```python
from build123d import *

# Parameters (mm, degrees)
SKETCH1_R           = 32.5
BOSS_EXTRUDE1_DEPTH = 6
SKETCH16_R          = 1
CUT_EXTRUDE8_DEPTH  = 7
SKETCH17_R          = 2
CUT_EXTRUDE9_DEPTH  = 2.4
SKETCH18_R          = 4.5
CUT_EXTRUDE10_DEPTH = 7
SKETCH19_R          = 1.65
CUT_EXTRUDE11_DEPTH = 10
CUT_EXTRUDE12_DEPTH = 3
CUT_EXTRUDE13_DEPTH = 7


with BuildPart() as part:
    # Sketch1 → Boss-Extrude1 (new body)
    with BuildSketch(Plane.XY):
        Circle(SKETCH1_R)
    extrude(amount=BOSS_EXTRUDE1_DEPTH)

    # Sketch16 → Cut-Extrude8 (cut, through all)
    with BuildSketch(Plane.XY.offset(6)):
        with Locations((-8, 0)):
            Circle(SKETCH16_R)
        with Locations((-5.656854249, 5.656854249)):
            Circle(SKETCH16_R)
        with Locations((0, 8)):
            Circle(SKETCH16_R)
        with Locations((5.656854249, 5.656854249)):
            Circle(SKETCH16_R)
        with Locations((8, 0)):
            Circle(SKETCH16_R)
        with Locations((5.656854249, -5.656854249)):
            Circle(SKETCH16_R)
        with Locations((0, -8)):
            Circle(SKETCH16_R)
        with Locations((-5.656854249, -5.656854249)):
            Circle(SKETCH16_R)
    extrude(amount=-CUT_EXTRUDE8_DEPTH, mode=Mode.SUBTRACT)

    # Sketch17 → Cut-Extrude9 (cut)
    with BuildSketch(Plane.XY.offset(6)):
        with Locations((7.5, 0)):
            Circle(SKETCH17_R)
        with Locations((-8, 0)):
            Circle(SKETCH17_R)
        with Locations((0, -7.5)):
            Circle(SKETCH17_R)
        with Locations((0, 7.5)):
            Circle(SKETCH17_R)
        with Locations((-5.656854249, 5.656854249)):
            Circle(SKETCH17_R)
        with Locations((5.656854249, 5.656854249)):
            Circle(SKETCH17_R)
        with Locations((5.656854249, -5.656854249)):
            Circle(SKETCH17_R)
        with Locations((-5.656854249, -5.656854249)):
            Circle(SKETCH17_R)
    extrude(amount=-CUT_EXTRUDE9_DEPTH, mode=Mode.SUBTRACT)

    # Sketch18 → Cut-Extrude10 (cut, through all)
    with BuildSketch(Plane(origin=(0, 0, 0), x_dir=(-1, 0, 0), z_dir=(0, 0, -1))):
        Circle(SKETCH18_R)
    extrude(amount=-CUT_EXTRUDE10_DEPTH, mode=Mode.SUBTRACT)

    # Sketch19 → Cut-Extrude11 (cut)
    with BuildSketch(Plane.XY.offset(6)):
        with Locations((0, 28)):
            Circle(SKETCH19_R)
        with Locations((28, 0)):
            Circle(SKETCH19_R)
        with Locations((0, -28)):
            Circle(SKETCH19_R)
        with Locations((-28, 0)):
            Circle(SKETCH19_R)
    extrude(amount=-CUT_EXTRUDE11_DEPTH, mode=Mode.SUBTRACT)

    # Sketch20 → Cut-Extrude12 (cut)
    with BuildSketch(Plane(origin=(0, 0, 0), x_dir=(-1, 0, 0), z_dir=(0, 0, -1))):
        Polygon((1.616580754, 30.8), (-1.616580754, 30.8), (-3.233161507, 28), (-1.616580754, 25.2), (1.616580754, 25.2), (3.233161507, 28), align=None)
        Polygon((29.616580754, 2.8), (26.383419246, 2.8), (24.766838493, 0), (26.383419246, -2.8), (29.616580754, -2.8), (31.233161507, 0), align=None)
        Polygon((1.616580754, -25.2), (-1.616580754, -25.2), (-3.233161507, -28), (-1.616580754, -30.8), (1.616580754, -30.8), (3.233161507, -28), align=None)
        Polygon((-26.383419246, 2.8), (-29.616580754, 2.8), (-31.233161507, 0), (-29.616580754, -2.8), (-26.383419246, -2.8), (-24.766838493, 0), align=None)
    extrude(amount=-CUT_EXTRUDE12_DEPTH, mode=Mode.SUBTRACT)

    # Sketch21 → Cut-Extrude13 (cut, through all)
    with BuildSketch(Plane.XY.offset(6)):
        with BuildLine():
            ThreePointArc((12.855752194, -15.320888862), (0, 20), (-12.855752194, -15.320888862))
            ThreePointArc((-12.855752194, -15.320888862), (-8.629256035, -14.951118362), (-8.999026536, -10.724622204))
            ThreePointArc((-8.999026536, -10.724622204), (0, 14), (8.999026536, -10.724622204))
            ThreePointArc((8.999026536, -10.724622204), (8.629256035, -14.951118362), (12.855752194, -15.320888862))
        make_face()
    extrude(amount=-CUT_EXTRUDE13_DEPTH, mode=Mode.SUBTRACT)


solid = part.part
```
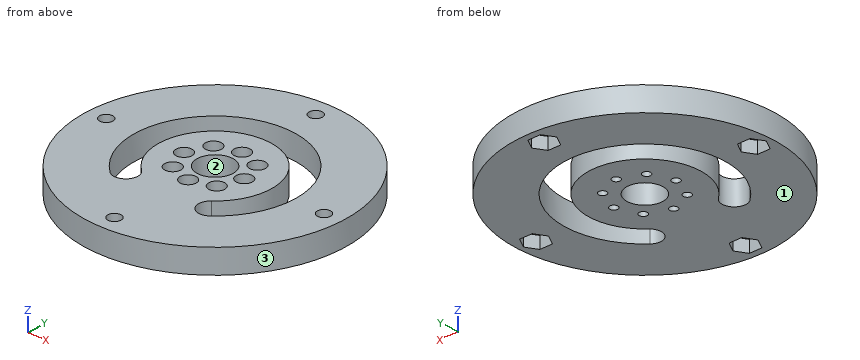
CAD build for the part. Positions are in the model's coordinates, mm. Face numbers are marked on the shaded views. Round coordinates to 2 decimals unless told otherwise and drop trailing zeros. Loops run counter-clockwise (first coordinate to the right, second up) from the corner with the lowest first, then second, coordinate; pieces in that order, holes last. Notation, with made-up numbers: (66.5, 24.25) - (77.5, 24.25) arc R19 cw to (77.5, 42.25) - close; hole circle Ø6 at (-12.75, -2). An arc over 180 degrees is marked (long way). Return JSON: item names as keys, results as strings. Group by question number.
Q1. Band-saw the part on B-B on y = -14. Give the cut face in (x, z).
Q2. Drill centre lines: line 1 along X through (y, z) = (-7.5, 0.85); line 2 along X through (y, z) = (-13, 1.8); line 3 along Y through (x, z) = (-11, 5.8). Where is each one in solid material? Low to high. Write a range as [from, to].
Q3. Band-saw the part on A-A on x = -28. Give the cut face in (y, z), plus the area to 3 significant figures.
Q4. Band-saw the part on D-D on x = -15. Give the cut face in (y, z), plus the area to 3 significant figures.
Q5. Flat gauge pins, fed straight in: pin 1 Ø3 at (x, y) = (-0.5, -27.5) entering from -Z; pin 2 Ø4.5 at (x, y) = (0, -7.5) entering from +Z; pin 3 Ø2 at (y, z) = (-10.5, 2) entering from -X; pin 4 Ø1.2 at (x, y) = (-6.5, 5.5) entering from +Z. Where does each tip first touch, or does it go through?
Q6. Two-plate mould, pull along X, no slides. Class the marked faces 1, 2 and 3: +X half, -X half, draft (parallel to the pull), parting line (faces both ways), or undercut.
Q7. Band-saw the part on C-C on x = 0. Give the number of separate pieces and of enclosed holes in the cut face, plus the area to 3 significant figures.
Solutions:
{
 "1": {"outline": "(-29.33, 0) - (-14.28, 0) - (-14.28, 6) - (-29.33, 6) - close; (-8.09, 0) - (8.09, 0) - (8.09, 6) - (-8.09, 6) - close; (14.28, 0) - (29.33, 0) - (29.33, 6) - (14.28, 6) - close"},
 "2": {"line 1": "x = [-31.62, -18.54], [-11.82, -0.87], [0.87, 11.82], [18.54, 31.62]", "line 2": "x = [-29.79, -15.2], [-7.93, 7.93], [15.2, 29.79]", "line 3": "y = [-30.58, -16.02], [-8.66, 8.66], [16.7, 30.58]"},
 "3": {"outline": "(-16.5, 0) - (-2.8, 0) - (-2.8, 3) - (-1.65, 3) - (-1.65, 6) - (-16.5, 6) - close; (1.65, 3) - (2.8, 3) - (2.8, 0) - (16.5, 0) - (16.5, 6) - (1.65, 6) - close", "area": "171 mm^2"},
 "4": {"outline": "(-28.83, 0) - (-13.23, 0) - (-13.23, 6) - (-28.83, 6) - close; (13.23, 0) - (28.83, 0) - (28.83, 6) - (13.23, 6) - close", "area": "187 mm^2"},
 "5": {"pin 1": "stops at z = 3", "pin 2": "stops at z = 6", "pin 3": "stops at x = -31.08", "pin 4": "stops at z = 3.6"},
 "6": {"face 1": "draft", "face 2": "undercut", "face 3": "parting line"},
 "7": {"separate pieces": "7", "enclosed holes": "0", "area": "213 mm^2"}
}
